The model under review builds one solid part; all positions refer to its coordinate system, in mm. A direction names the side the tool comes from. Coordinates: 2 decimals unless noted, no trailing zeros. Order: outer loops, then holes, each group sorted by start corner. A loop starts at its lowest first (then second) coordinate and runs counter-clockwise, first axis right, second up. Notation, with made-up numbers: M 57,35.25 L 80,35.25 A18 ccw 80,66.25 Z; hole C 23.25,72 d8. An arc over 180 degrees is marked long. Answer in a Markdown table with one row per item.
Autodesk Inventor part; units mm, degrees
ref_plane "Work Plane1" through (5, 0, 0) normal (0, 0.5, 0.8660254) x (1, 0, 0)
ref_plane "YZ Plane" through (0, 0, 0) normal (1, 0, 0) x (0, 1, 0)
ref_plane "XZ Plane" through (0, 0, 0) normal (0, 1, 0) x (-1, 0, 0)
sketch "草图1" plane through (0, 0, 0) normal (0, 0, 1) x (1, 0, 0)
  line L0 (-1, 0) -> (10, 0)
  line L1 (10, 0) -> (10, 8)
  line L2 (10, 8) -> (0, 8)
  line L3 (0, 8) -> (0, 10)
  line L4 (0, 10) -> (-1, 10)
  line L5 (-1, 10) -> (-1, 0)
  line L6 (-3.2, 0) -> (12.2, 0)
  line L7 (0, -2) -> (0, 12)
  line L8 (0, 7.0798) -> (9.9654, 7.0798) construction
  line L9 (2.5, 8) -> (1.7263, 7.2263)
  line L10 (1.069, 7.1826) -> (0, 8)
  arc A0 (1.069, 7.1826) -> (1.7263, 7.2263) centre (1.3727, 7.5798) ccw
  dimension "d0" = 16
  dimension "d1" = 10
  dimension "d2" = 1
  dimension "d3" = 20
  dimension "d5" = 14.1596
  dimension "d6" = 0.5
  dimension "d7" = 45
  dimension "d8" = 2.5
revolve "轴承体" add sketch "草图1" angle 360 about axis through (-1, 0, 0) along (1, 0, 0)
sketch "草图2" plane through (-1, 0, 0) normal (-1, 0, 0) x (0, 0, 1)
  circle A0 centre (0, 0) radius 10
  line L0 (6.3509, 11) -> (12.7017, 0)
  line L1 (12.7017, 0) -> (6.3509, -11)
  line L2 (6.3509, -11) -> (-6.3509, -11)
  line L3 (-6.3509, -11) -> (-12.7017, 0)
  line L4 (-12.7017, 0) -> (-6.3509, 11)
  line L5 (-6.3509, 11) -> (6.3509, 11)
  dimension "d11" = 22
extrude "头" add sketch "草图2" along normal blind 7 contours A0 | L0 L1 L2 L3 L4 L5
revolve "沟槽1" cut sketch "草图1" angle 360 about axis through (-1, 0, 0) along (1, 0, 0) contours L2 L9 A0 L10
sketch "草图3" plane through (0, 0, 0) normal (0, 1, 0) x (-1, 0, 0)
  line L0 (7.0175, 12.7017) -> (8, 12.7017)
  line L1 (8, 12.7017) -> (8, 11)
  line L2 (8, 11) -> (7.0175, 12.7017)
  line L3 (9.4, 0) -> (-0.4, 0)
  line L4 (1, 12.7017) -> (8, 12.7017)
  line L5 (8, 6.3509) -> (8, 12.7017)
  dimension "d14" = 30
  dimension "d15" = 11
revolve "倒角2" cut sketch "草图3" angle 360 about axis through (-10, 0, 0) along (1, 0, 0)
thread "螺纹"
chamfer "倒角1" distance 0.9202 distance2 2.5 1 edges at (10, -8, 0) measured on face at (10, -0.1598, -1.3157)
ref_plane "Work Plane1" through (5, 0, 0) normal (0, 0.5, 0.8660254) x (1, 0, 0)
equation "\"d11\" = SW"
equation "\"d12\" = KOH"
equation "\"d0\" = NND"
equation "\"d1\" = NLG"
equation "\"d2\" = SD"
equation "\"d3\" = SD2"
equation "\"d5\" = GD1"
equation "\"d6\" = 0.2 * GAL1"
equation "\"d8\" = GAL1"
equation "\"d17\" = GEL"
equation "\"d9\" = -0.5 * GD1 + 0.5 * NND"
equation "\"d10\" = GAL1"
equation "\"d15\" = 0.5 * SW"
equation "\"NND\" = 16"
equation "\"NLG\" = 10"
equation "\"GAL1\" = 2.5"
equation "\"SD\" = 1"
equation "\"SD2\" = 20"
equation "\"GD1\" = THREADDIA - 1.2269 * PTC"
equation "\"SW\" = 22"
equation "\"KOH\" = 7"
equation "\"GEL\" = NLG"
equation "\"GUL\" = 0.61345 * PTC"
equation "\"PHH\" = 0.8"
equation "\"RR\" = 1"
equation "\"THREADDIA\" = 16"
equation "\"TOA\" = 30deg"
equation "\"PTC\" = 1.5"
equation "\"GAL\" = 0.61345 * PTC"
equation "\"E0\" = 25.4"
properties part number "CSN 02 1915.11 - M16 x 1.5 x 10" material "钢，软"
(1) Machinability: for faces 1 (the flat face through (-1, 5.8, 8.4)), 2 (the conical face through (-7.76, 9.9, 5.68)), which of the approach directions +Z, -Z, +X, -X, +Y, -Y give a long, thin tool a straight path to every point of the face, cutting with its end or side? Answer none if there is none.
Report:
| item | result |
|---|---|
| face 1 | +X |
| face 2 | +Z, -X, +Y |
(2) Take a section at A-A (x = -5). Write out the cut boundary in (y, z), then the cut area to 3 significant figures.
Report:
| item | result |
|---|---|
| outline | M -11,-6.35 L 0,-12.7 L 11,-6.35 L 11,6.35 L 0,12.7 L -11,6.35 Z |
| area | 419 mm^2 |
(3) Insertion check: P1, Ø5, axis at x = 3, z = -2.5, coming from the -Y side; P2, Ø3, axis at x = 8, y = 8, coming from the +Z side; P3, Ø6, axis at x = 5, y = 8, coming from the +Z side (3 decimals). Each pin has a flat end and moves straight along its axis. Give the tip position at first contact, or say it passes through.
Report:
| item | result |
|---|---|
| P1 | y = -8 |
| P2 | z = 4.54 |
| P3 | z = 6.245 |
(4) To check wall thickness, follow line 1 (X direction, y = 8.75, z = -1.75); line 2 (Z direction, x = 3.75, y = -0.25); line 3 (X direction, y = -1.25, z = -10.5). State the ranges of each line that lie inside material, in increasing order. Write a range as [from, to].
Report:
| item | result |
|---|---|
| line 1 | [-8, 0] |
| line 2 | [-8, 8] |
| line 3 | [-8, -1] |
